Input: part model. Units: mm. Frame: model coordinates. A direction names the side the tool comes from. Give positions to 0.01 mm unless a question says otherwise; leave off trailing zeros. Write each loop counter-clockwise with the first axis right and the second up, starting at its lowest first coordinate (ties: lowest second). Pieces come first, ordered by that corner, then holes.
```python
from build123d import *

# Parameters (mm, degrees)
SKETCH1_R           = 35
SKETCH1_R_2         = 30
BOSS_EXTRUDE2_DEPTH = 14
FILLET1_R           = 3
FILLET2_R           = 3
FILLET3_R           = 1
SKETCH2_R           = 2.5
CUT_EXTRUDE1_DEPTH  = 5
CIRPATTERN3_COUNT   = 8


with BuildPart() as part:
    # Sketch1 → Boss-Extrude2 (new body)
    # profile 1 of 2: a face of its own
    with BuildSketch(Plane.XY):
        with BuildLine():
            Line((-6.598630751, 37.422694614), (-8.335112528, 47.270772145))
            ThreePointArc((-8.335112528, 47.270772145), (-13.431792673, 46.082393011), (-18.368804754, 44.346217561))
            Line((-18.368804754, 44.346217561), (-25.426963042, 28.239503368))
            Line((-25.426963042, 28.239503368), (-31.127777683, 21.795904581))
            Line((-31.127777683, 21.795904581), (-39.319298126, 27.531668945))
            ThreePointArc((-39.319298126, 27.531668945), (-42.082884274, 23.087460908), (-44.346217561, 18.368804754))
            Line((-44.346217561, 18.368804754), (-37.947922321, 1.988766337))
            Line((-37.947922321, 1.988766337), (-37.422694614, -6.598630751))
            Line((-37.422694614, -6.598630751), (-47.270772145, -8.335112528))
            ThreePointArc((-47.270772145, -8.335112528), (-46.082393011, -13.431792673), (-44.346217561, -18.368804754))
            Line((-44.346217561, -18.368804754), (-28.239503368, -25.426963042))
            Line((-28.239503368, -25.426963042), (-21.795904581, -31.127777683))
            Line((-21.795904581, -31.127777683), (-27.531668945, -39.319298126))
            ThreePointArc((-27.531668945, -39.319298126), (-23.087460908, -42.082884274), (-18.368804754, -44.346217561))
            Line((-18.368804754, -44.346217561), (-1.988766337, -37.947922321))
            Line((-1.988766337, -37.947922321), (6.598630751, -37.422694614))
            Line((6.598630751, -37.422694614), (8.335112528, -47.270772145))
            ThreePointArc((8.335112528, -47.270772145), (13.431792673, -46.082393011), (18.368804754, -44.346217561))
            Line((18.368804754, -44.346217561), (25.426963042, -28.239503368))
            Line((25.426963042, -28.239503368), (31.127777683, -21.795904581))
            Line((31.127777683, -21.795904581), (39.319298126, -27.531668945))
            ThreePointArc((39.319298126, -27.531668945), (42.082884274, -23.087460908), (44.346217561, -18.368804754))
            Line((44.346217561, -18.368804754), (37.947922321, -1.988766337))
            Line((37.947922321, -1.988766337), (37.422694614, 6.598630751))
            Line((37.422694614, 6.598630751), (47.270772145, 8.335112528))
            ThreePointArc((47.270772145, 8.335112528), (46.082393011, 13.431792673), (44.346217561, 18.368804754))
            Line((44.346217561, 18.368804754), (28.239503368, 25.426963042))
            Line((28.239503368, 25.426963042), (21.795904581, 31.127777683))
            Line((21.795904581, 31.127777683), (27.531668945, 39.319298126))
            ThreePointArc((27.531668945, 39.319298126), (23.087460908, 42.082884274), (18.368804754, 44.346217561))
            Line((18.368804754, 44.346217561), (1.988766337, 37.947922321))
            Line((1.988766337, 37.947922321), (-6.598630751, 37.422694614))
        make_face()
        Circle(SKETCH1_R, mode=Mode.SUBTRACT)
    # profile 2 of 2: a face of its own
    with BuildSketch(Plane.XY):
        Circle(SKETCH1_R)
        Circle(SKETCH1_R_2, mode=Mode.SUBTRACT)
    extrude(amount=BOSS_EXTRUDE2_DEPTH)

    # Fillet1
    fillet1_edges = [part.edges().sort_by_distance(p)[0] for p in [
        (-18.368804754, 44.346217561, 7),
    ]]
    fillet(fillet1_edges, radius=FILLET1_R)

    # Fillet2
    fillet2_edges = [part.edges().sort_by_distance(p)[0] for p in [
        (44.346217561, -18.368804754, 7),
        (18.368804754, -44.346217561, 7),
        (-18.368804754, -44.346217561, 7),
        (-44.346217561, -18.368804754, 7),
        (-44.346217561, 18.368804754, 7),
        (18.368804754, 44.346217561, 7),
        (44.346217561, 18.368804754, 7),
    ]]
    fillet(fillet2_edges, radius=FILLET2_R)

    # Fillet3
    fillet3_edges = [part.edges().sort_by_distance(p)[0] for p in [
        (39.319298126, -27.531668945, 7),
        (8.335112528, -47.270772145, 7),
        (-27.531668945, -39.319298126, 7),
        (-47.270772145, -8.335112528, 7),
        (-39.319298126, 27.531668945, 7),
        (-8.335112528, 47.270772145, 7),
        (27.531668945, 39.319298126, 7),
        (47.270772145, 8.335112528, 7),
    ]]
    fillet(fillet3_edges, radius=FILLET3_R)

    # Sketch2 → Cut-Extrude1 (cut)
    with BuildSketch(Plane(origin=(0, 0, 0), x_dir=(0, 0, -1), z_dir=(0.8191520442889921, -0.5735764363510456, 0))):
        with Locations(Location((-3.5, 43, 0), (0, 0, 90))):
            Circle(SKETCH2_R)
        with Locations(Location((-10.5, 43, 0), (0, 0, 90))):
            Circle(SKETCH2_R)
    cut_extrude1 = extrude(amount=-CUT_EXTRUDE1_DEPTH, mode=Mode.SUBTRACT)

    # CirPattern3: Cut-Extrude1 ×8 about axis
    cirpattern3_axis = Axis((0, 0, 0), (0, 0, 1))
    for i in range(1, CIRPATTERN3_COUNT):
        add(cut_extrude1.rotate(cirpattern3_axis, i * 360 / CIRPATTERN3_COUNT), mode=Mode.SUBTRACT)


solid = part.part
```
Item 1: Section A-A (y = 0). Return loops of the section in (x, z).
Item 2: Mould query, pull axis Z, two halves, no side actions, for faces 1 (the flat face through (41.79, 7.37, 6.9)), 2 (the flat face through (-41.444, -12.385, 3.535)), 3 (the flat face through (-22, 22, 14)). Classes: +Z half, -Z half, draft (parallel to the pull), parting line (faces both ways), or undercut.
Item 3: Ray query, line 1 (Y direction, x = -22, z = 4.5); line 2 (Y direction, x = 20, z = 12); line 3 (X direction, y = 25, z = 8.5). Return the intervals inside material, ascending.
Item 4: Set-up query: faces 4 (the cylindrical face through (23.247, 41.995, 6.902)), 5 (the flat face through (-37.69, -2.24, 6.9)), 6 (the flat face through (20.548, 38.063, 10.535)). Return all of +Z, -Z, +X, -X, +Y, -Y with unobstructed straight access to the full face (end or side cutting, diameter ignored); none if empty.
Item 5: Pin query (flat end, axial travel): pin 1 (8 mm diameter, centred on x = -8, z = 3, fed in from -Y); pin 2 (6 mm diameter, centred on x = 34.5, z = 2, fed in from -Y). Return the tip coordinate at first contact, or that it passes through.
Solved:
1. outline: (-37.83, 0) - (-30, 0) - (-30, 14) - (-37.83, 14) - close; (30, 0) - (37.83, 0) - (37.83, 14) - (30, 14) - close
2. face 1: draft
2. face 2: undercut
2. face 3: +Z half
3. line 1: y = -42.66 to -39.89, -34.29 to -31.42, -30.95 to -20.4, 20.4 to 36.06
3. line 2: y = -40.62 to -22.36, 22.36 to 36.05, 37.28 to 43.63
3. line 3: x = -40.98 to -36.82, -28.29 to -16.58, 16.58 to 29.21
4. face 4: +Z, -Z, +X, +Y
4. face 5: +Z, -Z, -X
4. face 6: none
5. pin 1: stops at y = -41.86
5. pin 2: stops at y = -26.26
